Autodesk Inventor part; units mm, degrees
ref_plane "YZ Plane" through (0, 0, 0) normal (1, 0, 0) x (0, 1, 0)
ref_plane "XZ Plane" through (0, 0, 0) normal (0, 1, 0) x (-1, 0, 0)
ref_plane "XY Plane" through (0, 0, 0) normal (0, 0, 1) x (1, 0, 0)
sketch "Sketch1" plane through (0, 0, 0) normal (1, 0, 0) x (0, 1, 0)
  line L0 (7.5, 0) -> (-7.5, 0)
  line L1 (-7.5, 0) -> (-7.5, -15)
  line L2 (-7.5, -15) -> (-13.5, -15)
  circle A0 centre (0, 46.081) radius 11.15
  line L3 (7.5, 0) -> (7.5, -15)
  line L4 (7.5, -15) -> (13.5, -15)
  line L5 (-13.5, -15) -> (-13.5, 56.0455)
  line L6 (-13.5, 56.0455) -> (-9.9645, 59.581)
  line L7 (-9.9645, 59.581) -> (9.9645, 59.581)
  line L8 (9.9645, 59.581) -> (13.5, 56.0455)
  line L9 (13.5, 56.0455) -> (13.5, -15)
  point P0 (0, 0)
  point P1 (0, 0)
  point P2 (-13.5, 20.5227)
  dimension "d0" = 15
  dimension "d1" = 46.081
  dimension "d2" = 22.3
  dimension "d9" = 45
  dimension "d10" = 13.5
  dimension "d11" = 5
  dimension "d12" = 27
extrude "Extrusion1" add sketch "Sketch1" along normal blind 9
sketch "Sketch2" plane through (0, 0, 0) normal (-1, 0, 0) x (0, 0, 1)
  circle A0 centre (46.081, 0) radius 11.15
  circle A1 centre (46.081, 0) radius 9.15
  point P0 (0, 0)
  dimension "d13" = 2
extrude "Extrusion2" add sketch "Sketch2" against normal blind 2
sketch "Sketch3" plane through (0, 0, 0) normal (-1, 0, 0) x (0, 0, 1)
  circle A0 centre (46.081, 0) radius 9.15
  line L0 (-15, 13.5) -> (56.0455, 13.5)
  line L1 (-15, 7.5) -> (-15, 13.5)
  line L2 (0, 7.5) -> (-15, 7.5)
  line L3 (0, -7.5) -> (0, 7.5)
  line L4 (-15, -7.5) -> (0, -7.5)
  line L5 (-15, -13.5) -> (-15, -7.5)
  line L6 (56.0455, -13.5) -> (-15, -13.5)
  line L7 (59.581, -9.9645) -> (56.0455, -13.5)
  line L8 (59.581, 9.9645) -> (59.581, -9.9645)
  line L9 (56.0455, 13.5) -> (59.581, 9.9645)
  line L10 (-15, -13.5) -> (-15, -7.5)
  line L11 (-15, -13.5) -> (-15, -28.5)
  line L12 (-15, -28.5) -> (0, -28.5)
  line L13 (56.0455, -13.5) -> (-15, -13.5)
  line L14 (0, -28.5) -> (56.0455, -13.5)
  line L15 (-15, 13.5) -> (56.0455, 13.5)
  line L16 (56.0455, 13.5) -> (0, 28.5)
  line L17 (0, 28.5) -> (-15, 28.5)
  line L18 (-15, 28.5) -> (-15, 13.5)
  point P0 (0, 0)
  dimension "d16" = 15
  dimension "d17" = 15
extrude "Extrusion3" add sketch "Sketch3" against normal blind 4 contours L18 L17 L16 L0 | L14 L12 L11 L6
sketch "Sketch4" plane through (9, 0, 0) normal (1, 0, 0) x (0, 0, -1)
  line L0 (15, 13.5) -> (-56.0455, 13.5)
  line L1 (15, 7.5) -> (15, 13.5)
  line L2 (0, 7.5) -> (15, 7.5)
  line L3 (0, -7.5) -> (0, 7.5)
  line L4 (15, -7.5) -> (0, -7.5)
  line L5 (15, -13.5) -> (15, -7.5)
  line L6 (-56.0455, -13.5) -> (15, -13.5)
  line L7 (0, -7.5) -> (0, -13.5)
  line L8 (0, 7.5) -> (15, 7.5)
  line L9 (0, 7.5) -> (0, 13.5)
  point P0 (0, 0)
extrude "Extrusion4" add sketch "Sketch4" along normal blind 15
chamfer "Chamfer2" distance 2 distance2 15 1 edges at (9, 10.5, 0) measured on face at (9, 0.448, 11.6708)
sketch "Sketch5" plane through (24, 13.5, 0) normal (0, 1, 0) x (1, 0, 0)
  line L0 (0, 0) -> (-15, -2)
  line L1 (0, 15) -> (0, 0)
  line L2 (-20, 15) -> (0, 15)
  line L3 (-20, 15) -> (-20, -56.0455)
  line L4 (-20, -56.0455) -> (-15, -56.0455)
  line L5 (-15, -2) -> (-15, -56.0455)
  point P0 (-24, 0)
  point P1 (-10, 7.5)
  point P2 (-10, 15)
  point P3 (0, 7.5)
hole "Hole1" at (14, 13.5, -7.5) direction (0, -1, 0) diameter 3.6 end through all counterbore diameter 6.5 counterbore depth 3.4
sketch "Sketch7" plane through (4, 0, 0) normal (1, 0, 0) x (0, 0, -1)
  line L0 (15, 28.5) -> (0, 28.5)
  line L1 (0, 28.5) -> (-56.0455, 13.5)
  line L2 (15, 13.5) -> (-56.0455, 13.5)
  line L3 (15, 13.5) -> (15, 28.5)
  point P0 (0, 0)
  point P1 (7.5, 21)
  point P2 (7.5, 28.5)
  point P3 (15, 21)
hole "Hole3" at (4, 21, -7.5) direction (-1, 0, 0) diameter 3.6 end through all counterbore diameter 6.5 counterbore depth 1
mirror "Mirror1" about plane through (0, 0, 0) normal (0, 1, 0) of "Hole3", "Hole1"
chamfer "Chamfer6" distance 5 angle 45 2 edges at (4, 13.5, 20.5227) (4, -13.5, 20.5227)
properties part number "Rear Z Axis Top Bearing" material "ABS Plastic"
Design review of the part built by this model. Coordinates are the model's own, in mm. A direction names the side the tool comes from. Give positions to 0.01 mm unless a question says otherwise; leave off trailing zeros. Loops run counter-clockwise (first coordinate to the right, second up) from the corner with the lowest first, then second, coordinate; pieces in that order, holes last. Notation, with made-up numbers: (-1, 54.25) -> (8, 54.25) arc R24 ccw to (8, 92.25) -> close; hole circle Ø8 at (40, 72). An arc over 180 degrees is marked (long way). One line per question, with ' | ' between items. Start each with the question number.
(1) For faces 4 (the face through (16, -10, 0)), 5 (the face through (4, -22, 5)), 6 (the face through (3.474, -17.827, -6.795)), list the 3-axis set-ups (+Z, -Z, +X, -X, +Y, -Y) from which the entire face can be reached by the end or side of a thin tool; tool diameter is ignored.
(2) Insertion check: P1, Ø10.5, axis at x = 14, z = -7.5, coming from the +Y side; P2, Ø12, axis at y = -16.5, z = 21.5, coming from the +X side; P3, Ø6, axis at y = 18, z = 47.5, coming from the -X side; P4, Ø8.5, axis at y = -21, z = -7.5, coming from the +X side. Each pin has a flat end and moves straight along its axis. Give the tip position at first contact, or say it passes through.
(3) Draft analysis for pull direction Y (two halves, no side actions). For faces 1 (the face through (6.5, -16, 13.1)), 2 (the face through (1.479, 19.215, -7.266)), 3 (the face through (9, 0, 24)), state which applies: +Y half, -Y half, draft (parallel to the pull), parting line (faces both ways), or undercut.
(4) We need section A-A (z = 48). State the section outline as (x, y) points, and give its area (3 significant figures).
(5) We need section C-C (x = 14). State the section outline as (y, z) points, and give its area (3 significant figures).
(6) We need section B-B (y = 0). State the section outline as (x, z) points.
(7) We need section D-D (x = 19). State the section outline as (y, z) points.
(8) For line 1 (Y direction, x = 0.65, z = -7.5); line 2 (X direction, y = 12.8, z = -7.5); line 3 (Z direction, x = 14, y = -8.55), list the stretches that pass through material, from the lowest coordinate up.
The answers:
1) face 4: +Z, +X, -Y | face 5: +Z, -Z, +X, -Y | face 6: +X
2) P1: stops at y = 13.75 | P2: stops at x = 9 | P3: stops at x = 0 | P4: stops at x = 5.75
3) face 1: -Y half | face 2: undercut | face 3: draft
4) outline: (0, -15.65) -> (6.85, -15.65) -> (9, -13.5) -> (9, -10.98) -> (2, -10.98) -> (2, -8.95) -> (0, -8.95) -> close; (0, 8.95) -> (2, 8.95) -> (2, 10.98) -> (9, 10.98) -> (9, 13.5) -> (6.85, 15.65) -> (0, 15.65) -> close | area: 87.6 mm^2
5) outline: (-13.5, -15) -> (-7.5, -15) -> (-7.5, -9.3) -> (-10.1, -9.3) -> (-10.1, -10.75) -> (-13.5, -10.75) -> close; (-13.5, -4.25) -> (-10.1, -4.25) -> (-10.1, -5.7) -> (-7.5, -5.7) -> (-7.5, 0) -> (-13.5, 0) -> close; (7.5, -15) -> (13.5, -15) -> (13.5, -10.75) -> (10.1, -10.75) -> (10.1, -9.3) -> (7.5, -9.3) -> close; (7.5, -5.7) -> (10.1, -5.7) -> (10.1, -4.25) -> (13.5, -4.25) -> (13.5, 1.33) -> (7.5, 1.33) -> close | area: 125 mm^2
6) outline: (0, 0) -> (9, 0) -> (9, 34.93) -> (2, 34.93) -> (2, 36.93) -> (0, 36.93) -> close; (0, 55.23) -> (2, 55.23) -> (2, 57.23) -> (9, 57.23) -> (9, 59.58) -> (0, 59.58) -> close
7) outline: (-13.5, -15) -> (-7.5, -15) -> (-7.5, 0) -> (-13.5, 0) -> close; (7.5, -15) -> (13.5, -15) -> (13.5, 0.67) -> (7.5, 0.67) -> close
8) line 1: y = -28.5 to -22.8, -19.2 to -7.5, 7.5 to 19.2, 22.8 to 28.5 | line 2: x = 0 to 10.75, 17.25 to 24 | line 3: z = -15 to -9.3, -5.7 to 0
